from build123d import *

# Parameters (mm, degrees)
SKETCH1_W           = 139
SKETCH1_H           = 86
SKETCH1_R           = 1.6
SKETCH1_R_2         = 3.1
SKETCH1_R_3         = 1.25
SKETCH1_W_2         = 2.7
SKETCH1_H_2         = 1.2
SKETCH1_H_3         = 1.309440744
BOSS_EXTRUDE1_DEPTH = 3


with BuildPart() as part:
    # Sketch1 → Boss-Extrude1 (new body)
    with BuildSketch(Plane.XY):
        with Locations((69.5, 43)):
            Rectangle(SKETCH1_W, SKETCH1_H)
        with Locations((4, 58.5)):
            Circle(SKETCH1_R, mode=Mode.SUBTRACT)
        with Locations((135, 58.5)):
            Circle(SKETCH1_R, mode=Mode.SUBTRACT)
        with Locations((135, 14.5)):
            Circle(SKETCH1_R, mode=Mode.SUBTRACT)
        with Locations((4, 14.5)):
            Circle(SKETCH1_R, mode=Mode.SUBTRACT)
        with Locations((49.136550625, 30.80578632)):
            Circle(SKETCH1_R, mode=Mode.SUBTRACT)
        with Locations((119, 30.80578632)):
            Circle(SKETCH1_R, mode=Mode.SUBTRACT)
        with Locations((56.141769292, 62)):
            Circle(SKETCH1_R_2, mode=Mode.SUBTRACT)
        with Locations((28.227965057, 11.99453943)):
            Circle(SKETCH1_R_2, mode=Mode.SUBTRACT)
        with Locations((111.806450526, 68.419506212)):
            Circle(SKETCH1_R_2, mode=Mode.SUBTRACT)
        with Locations((84.154646153, 68.419506212)):
            Circle(SKETCH1_R_2, mode=Mode.SUBTRACT)
        with Locations((135, 80.5)):
            Circle(SKETCH1_R_3, mode=Mode.SUBTRACT)
        with Locations((4, 80.5)):
            Circle(SKETCH1_R_3, mode=Mode.SUBTRACT)
        with Locations((28.227965057, 68.419506212)):
            Circle(SKETCH1_R_2, mode=Mode.SUBTRACT)
        with Locations((28.227965057, 33.99453943)):
            Circle(SKETCH1_R_2, mode=Mode.SUBTRACT)
        with Locations((28.227965057, 5.99453943)):
            Rectangle(SKETCH1_W_2, SKETCH1_H_2, mode=Mode.SUBTRACT)
        with Locations((84.154646153, 62.419506212)):
            Rectangle(SKETCH1_W_2, SKETCH1_H_2, mode=Mode.SUBTRACT)
        with Locations((56.141769292, 56)):
            Rectangle(SKETCH1_W_2, SKETCH1_H_2, mode=Mode.SUBTRACT)
        with Locations((111.806450526, 62.419506212)):
            Rectangle(SKETCH1_W_2, SKETCH1_H_2, mode=Mode.SUBTRACT)
        with Locations((28.227965057, 62.419506212)):
            Rectangle(SKETCH1_W_2, SKETCH1_H_2, mode=Mode.SUBTRACT)
        with Locations((28.227965057, 27.99453943)):
            Rectangle(SKETCH1_W_2, SKETCH1_H_3, mode=Mode.SUBTRACT)
    extrude(amount=BOSS_EXTRUDE1_DEPTH)


solid = part.part
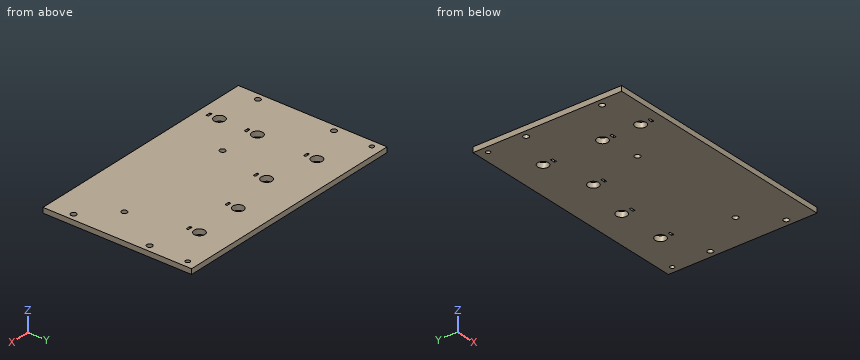
Design review of the part built by this model. Coordinates are the model's own, in mm. Round coordinates to 2 decimals unless told otherwise and drop trailing zeros. Write each loop counter-clockwise with the first axis right and the second up, starting at its lowest first coordinate (ties: lowest second). Pieces come first, ordered by that corner, then holes. Notation, with made-up numbers: (-39, 64) - (-20, 64) arc R21 ccw to (-20, 68) - close; hole circle Ø6 at (78.5, -32). An arc over 180 degrees is marked (long way). Use a Markdown table: item, result. Add a question column.
1. We need section A-A (x = 119). State the section outline as (y, z) points, then the cut area to 3 significant figures.
2. We need section B-B (z = 1.6). Count the separate pieces of the cut face and the enclosed holes in it, then the cut area to 3 significant figures.
3. Wall thickness on probe 1 along Y at (x, z) = (4, 0.9); probe 2 along X at (y, z) = (81, 1.5); probe 3 along X at (y, z) = (69.5, 0.5): over which ranges is each line inside the solid? List them lowest first.
Output:
| question | item | result |
|---|---|---|
| 1 | outline | (0, 0) - (29.21, 0) - (29.21, 3) - (0, 3) - close; (32.41, 0) - (86, 0) - (86, 3) - (32.41, 3) - close |
| 1 | area | 248 mm2 |
| 2 | separate pieces | 1 |
| 2 | enclosed holes | 20 |
| 2 | area | 11,700 mm2 |
| 3 | probe 1 | y = 0 to 12.9, 16.1 to 56.9, 60.1 to 79.25, 81.75 to 86 |
| 3 | probe 2 | x = 0 to 2.85, 5.15 to 133.85, 136.15 to 139 |
| 3 | probe 3 | x = 0 to 25.32, 31.13 to 81.25, 87.06 to 108.9, 114.71 to 139 |
